Autodesk Fusion 360 part; units mm, degrees
sketch "Sketch1" plane through (0, 0, 0) normal (0, 0, 1) x (1, 0, 0)
  line L0 (0, 0) -> (50, 0)
  line L1 (50, 8) -> (50, 10)
  line L2 (40, 10) -> (0, 10)
  line L3 (0, 10) -> (0, 0)
  line L4 (50, 10) -> (40, 10) construction
  line L5 (50, 10) -> (50, 12)
  line L6 (50, 12) -> (40, 12)
  line L7 (40, 12) -> (40, 10)
  line L8 (50, 0) -> (57, 0) construction
  arc A0 (70.8924, 0) -> (50, 12) centre (57, 0) ccw
  arc A1 (69.2066, 0) -> (50, 10) centre (57, 0) ccw
  line L9 (50, 0) -> (70.8924, 0)
  line L10 (0, 0) -> (0, 8) construction
  line L11 (0, 8) -> (50, 8)
  line L12 (50, 8) -> (50, 10)
  dimension "d1" = 50
  dimension "d2" = 10
  dimension "d3" = 10
  dimension "d4" = 10
  dimension "d5" = 2
  dimension "d6" = 7
  dimension "d7" = 8
  dimension "d8" = 50
revolve "Revolve1" add sketch "Sketch1" angle 360 about axis through (0, 0, 0) along (1, 0, 0) contours L1 L2 L3 L5 L6 L7 L11 L12 | L5 A0 A1 L9
Part model, mm, in its own coordinate system. A direction names the side the tool comes from. Coordinates: 2 decimals unless noted, no trailing zeros. Loops run counter-clockwise (first coordinate to the right, second up) from the corner with the lowest first, then second, coordinate; pieces in that order, holes last. Notation, with made-up numbers: (-10.75, -17) - (40.25, -17) arc R23 cw to (40.25, -3) - close; hole circle Ø1 at (35, 60). An arc over 180 degrees is marked (long way). Write item = value, one per line. Start each with the question number.
Item 1: Cut at B-B, the plane x = 33.5. Give the cut face in (y, z).
Item 2: Cut at A-A, the plane x = 44. Give the cut face in (y, z).
Item 3: Wall check: L1, parallel to Z at x = 28, y = 0; L2, parallel to Z at x = 44.5, y = 1.5; L3, parallel to X at y = -1.5, z = -10.5. Give the ranges that are in metal, low to high. Write a range as from..to.
Item 4: Flat gauge pins, fed straight in: pin 1 Ø1 at (y, z) = (-10, 2.5) entering from +X; pin 2 Ø10 at (x, z) = (42, 9) entering from -Y; pin 3 Ø3 at (x, y) = (41.5, 0.5) entering from -Z. Where does each tip first touch, or does it go through?
Item 5: 3-axis set-ups, long thin cutter, end or side, ignore diameter. For faces 5 (the cylindrical face through (19.72, -2.17, 9.76)), 6 (the flat face through (0, 0, 8.2)): which of +Z, -Z, +X, -X, +Y, -Y reach the whole face in a straight line?
Item 6: Mould opens along Z. For faces 1 (the flat face through (40, -5, 9)), 2 (the cylindrical face through (44.93, -11.99, -0.53)), 3 (the cylindrical face through (25.35, -1.73, -7.81)), 4 (the flat face through (50, 0, 8.2)) say: released by +Z, released by -Z, zero draft, split by the parting line, or undercut.
The answers:
q1.outline = circle Ø20 at (0, 0); hole circle Ø16 at (0, 0)
q2.outline = circle Ø24 at (0, 0); hole circle Ø16 at (0, 0)
q3.L1 = -10..-8, 8..10
q3.L2 = -11.91..-7.86, 7.86..11.91
q3.L3 = 40..50.96, 63.04..65.97
q4.pin_1 = 66.84
q4.pin_2 = -11.31
q4.pin_3 = -12
q5.face_5 = -X
q5.face_6 = +Z, -Z, -X, +Y, -Y
q6.face_1 = zero draft
q6.face_2 = split by the parting line
q6.face_3 = undercut
q6.face_4 = undercut
